Build history of the part. All positions in model axes, mm. Round coordinates to 2 decimals unless told otherwise and drop trailing zeros. Write each loop counter-clockwise with the first axis right and the second up, starting at its lowest first coordinate (ties: lowest second). Pieces come first, ordered by that corner, then holes. Notation, with made-up numbers: (13, 23.25) -> (50, 23.25) arc R23 cw to (50, 44.25) -> close; hole circle Ø2 at (41, 89). An arc over 180 degrees is marked (long way). One line per question, with ' | ' between items.
from build123d import *

# Parameters (mm, degrees)
F0_R     = 25.4
F1_DEPTH = 101.6
F2_DEPTH = 101.854


with BuildPart() as f1:
    # F0 (on Top) → F1 (new body)
    with BuildSketch(Plane.XY):
        Polygon((1574.8, 0), (0, 0), (0, -50.8), (201.6062499031, -76.2), (1373.1937500969, -76.2), (1574.8, -50.8), (1574.8, -26.67), align=None)
        with Locations((1549.4, -26.67)):
            Circle(F0_R, mode=Mode.SUBTRACT)
        with Locations((1549.4, -26.67)):
            Circle(F0_R)
    extrude(amount=F1_DEPTH)

    # F0 (on Top) → F2 (join)
    with BuildSketch(Plane.XY):
        with Locations((1549.4, -26.67)):
            Circle(F0_R)
    extrude(amount=F2_DEPTH)


solid = f1.part
(1) Slice it at C-C (x = 174.5). Write the cut outline in (y, z).
Calculated:
outline: (-72.78, 0) -> (0, 0) -> (0, 101.6) -> (-72.78, 101.6) -> close
(2) Slice it at A-A (x = 1549.4). Write the cut outline in (y, z).
Calculated:
outline: (-54, 0) -> (0, 0) -> (0, 101.6) -> (-1.27, 101.6) -> (-1.27, 101.85) -> (-52.07, 101.85) -> (-52.07, 101.6) -> (-54, 101.6) -> close
(3) Wall check: line 1 (Z direction, x = 577.5, y = -41); line 2 (Y direction, x = 1485, z = 12). Give the ranges that are in metal, low to high. Write a range as from..to.
Calculated:
line 1: 0..101.6 | line 2: -62.11..0
(4) Slice it at B-B (z = 39). Write the cut outline in (x, y), then the cut area to 3 significant figures.
Calculated:
outline: (0, -50.8) -> (201.61, -76.2) -> (1373.19, -76.2) -> (1574.8, -50.8) -> (1574.8, 0) -> (0, 0) -> close | area: 115,000 mm2
(5) Drop a flat-ended pin along its axis: pin 1 (6 mm diameter, centred on x = 993, y = -32, fed in from +Z). Give the stop position or say it passes through.
Calculated:
pin 1: z = 101.6
